The figure shows three views and two pictorial views of one solid part (mm, origin at its lowest corner). Answer the questions. A direction names the side the tool comes from. Coordinates: 2 decimals unless noted, no trailing zeros. Write each loop counter-clockwise with the first axis right and the second up, starting at its lowest first coordinate (ties: lowest second). Pieces come first, ordered by that corner, then holes.
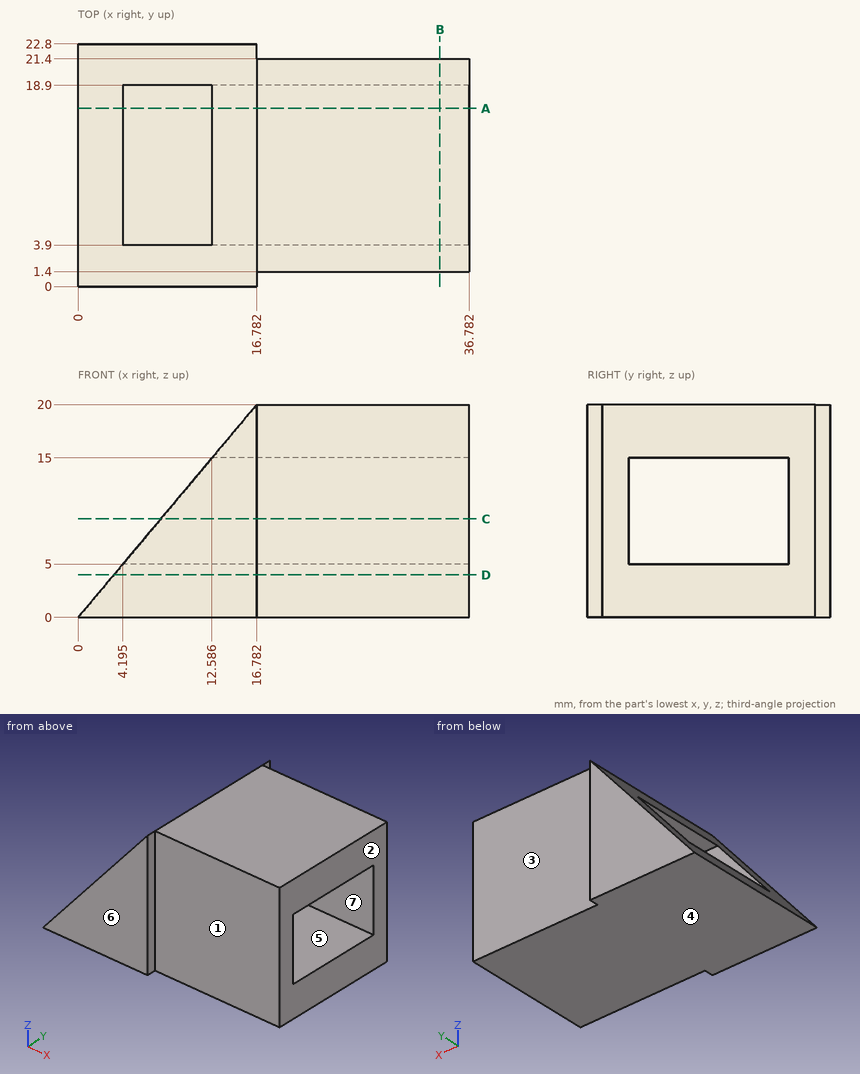
Q1. The part is cut by section C-C, the plane z = 9.25. Write down the section's boundary in (x, y).
Answers below:
outline: (7.76, 0) - (16.78, 0) - (16.78, 1.4) - (36.78, 1.4) - (36.78, 3.9) - (7.76, 3.9) - close; (7.76, 18.9) - (36.78, 18.9) - (36.78, 21.4) - (16.78, 21.4) - (16.78, 22.8) - (7.76, 22.8) - close
Q2. Determine the mould class of the marked faces 4, 5, 6 and 7 for opening direction Z: released by +Z, released by -Z, zero draft, split by the parting line, or undercut.
Answers below:
face 4: released by -Z
face 5: undercut
face 6: zero draft
face 7: undercut
Q3. The part is cut by section A-A, the plane y = 16.75. Write down the section's boundary in (x, z) (1 decimal).
Answers below:
outline: (0, 0) - (36.8, 0) - (36.8, 5) - (4.2, 5) - close; (12.6, 15) - (36.8, 15) - (36.8, 20) - (16.8, 20) - close
Q4. The part is cut by section B-B, the plane x = 34. Write down the section's boundary in (y, z), then the cut area to 3 significant figures.
Answers below:
outline: (1.4, 0) - (21.4, 0) - (21.4, 20) - (1.4, 20) - close; hole (3.9, 5) - (18.9, 5) - (18.9, 15) - (3.9, 15) - close
area: 250 mm2
Q5. Given pin 1 (8 mm diameter, centred on x = 23, z = 9, fed in from -Y); pin 2 (12 mm diameter, centred on y = 3.5, z = 4, fed in from -X); pin 3 (1.5 mm diameter, centred on y = 22.5, z = 9.5, fed in from +X); pin 4 (6 mm diameter, centred on x = 25, z = 12, fed in from +Y), each flat-ended and moving along its own axis, determine where each tip first touches the part or whether it passes through.
Answers below:
pin 1: stops at y = 1.4
pin 2: stops at x = 0
pin 3: stops at x = 16.78
pin 4: stops at y = 21.4
Q6. Find the intervals of material crossed by probe 1 along Y at (x, z) = (10.5, 10.75); probe 2 along Y at (x, z) = (27, 7); probe 3 along Z at (x, y) = (18.5, 5.75), in increasing order.
Answers below:
probe 1: y = 0 to 3.9, 18.9 to 22.8
probe 2: y = 1.4 to 3.9, 18.9 to 21.4
probe 3: z = 0 to 5, 15 to 20
Q7. The part is cut by section D-D, the plane z = 4. Write down the section's boundary in (x, y).
Answers below:
outline: (3.36, 0) - (16.78, 0) - (16.78, 1.4) - (36.78, 1.4) - (36.78, 21.4) - (16.78, 21.4) - (16.78, 22.8) - (3.36, 22.8) - close
Q8. Which of the six approach directions +Z, -Z, +X, -X, +Y, -Y give full straight-line access (tool end or side, diameter ignored) to the marked faces 1, 2 and 3?
Answers below:
face 1: +Z, -Z, +X, -Y
face 2: +Z, -Z, +X, +Y, -Y
face 3: +Z, -Z, +X, +Y
